Geometry: see drawing. Coordinates: mm, zero at the bounding-box minimum. A direction names the side the tool comes from. Give positions to 0.01 mm unless a question says otherwise; leave off trailing zeros. Order: outer loops, then holes, each group sorted by start corner. A loop starts at its lowest first (then second) coordinate and runs counter-clockwise, first axis right, second up. Notation, with made-up numbers: (-21, 35.5) - (-16, 35.5) arc R36 cw to (-16, 71.5) - close; hole circle Ø6 at (4.25, -4.5). An arc over 180 degrees is marked (long way). One line per question, with ' | ' between items. Start each with the question number.
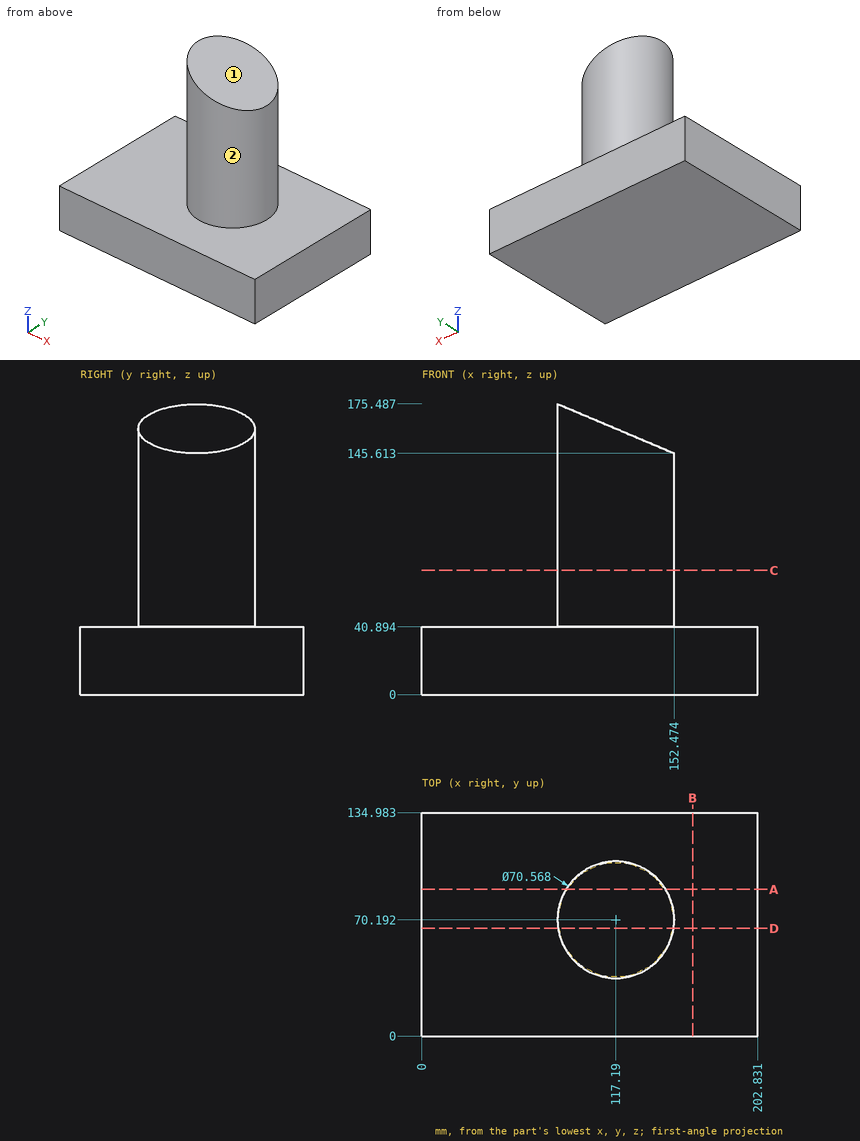
(1) Cut plane B-B, the plane x = 163.5. Return the cut outline in (y, z).
(2) Cut plane C-C, the plane z = 75. Return the cut outline in (x, y) (1 decimal), plus the area to 3 significant figures.
(3) Cut plane A-A, the plane y = 88.5. Return the cut outline in (x, z).
(4) Material intervals for line 1 along Z through (x, y) = (148, 110.5); line 2 along Y through (x, z) = (119, 129.5) (1 decimal); line 3 along Y through (x, z) = (137.5, 143) (1 decimal), sorted ascending. Write a range as from..to.
(5) Access query for the marked faces 1 and 2. Directions: +Z, -Z, +X, -X, +Y, -Y. A direction counts if a zero-diameter tool reaches every point of the face in a straight line with its end or side. Return the directions, or none.
(6) Cut plane D-D, the plane y = 65. Return the cut outline in (x, z) (1 decimal).
(7) Contact query for flat-ended pins moving along their axis: P1, Ø12, axis at y = 79.5, z = 141.5, coming from the -X side; P2, Ø2, axis at x = 94.5, z = 146, coming from the -Y side; P3, Ø1, axis at y = 58.5, z = 88, coming from the -X side. Output: stop coordinate, or through.
Results are:
1) outline: (0, 0) - (134.98, 0) - (134.98, 40.89) - (0, 40.89) - close
2) outline: circle Ø70.6 at (117.2, 70.2) | area: 3,910 mm2
3) outline: (0, 0) - (202.83, 0) - (202.83, 40.89) - (147.35, 40.89) - (147.35, 147.78) - (87.03, 173.32) - (87.03, 40.89) - (0, 40.89) - close
4) line 1: 0..40.89 | line 2: 35..105.4 | line 3: 41.3..99
5) face 1: +Z, +X, +Y, -Y | face 2: +Z
6) outline: (0, 0) - (202.8, 0) - (202.8, 40.9) - (152.1, 40.9) - (152.1, 145.8) - (82.3, 175.3) - (82.3, 40.9) - (0, 40.9) - close
7) P1: x = 82.06 | P2: y = 42.36 | P3: x = 83.73
